The drawing under review shows one solid part. Ordinate dimensions are in mm from its lowest x, y, z. A direction names the side the tool comes from. Give positions to 0.01 mm unless a question says otherwise; leave off trailing zeros. Loops run counter-clockwise (first coordinate to the right, second up) from the corner with the lowest first, then second, coordinate; pieces in that order, holes last. Notation, with made-up numbers: (5.25, 42) - (38.25, 42) arc R8 ccw to (38.25, 55) - close; hole circle Ø7 at (40, -17.5). An arc over 180 degrees is marked (long way). Return JSON: item names as keys, results as strings. Group by question number.
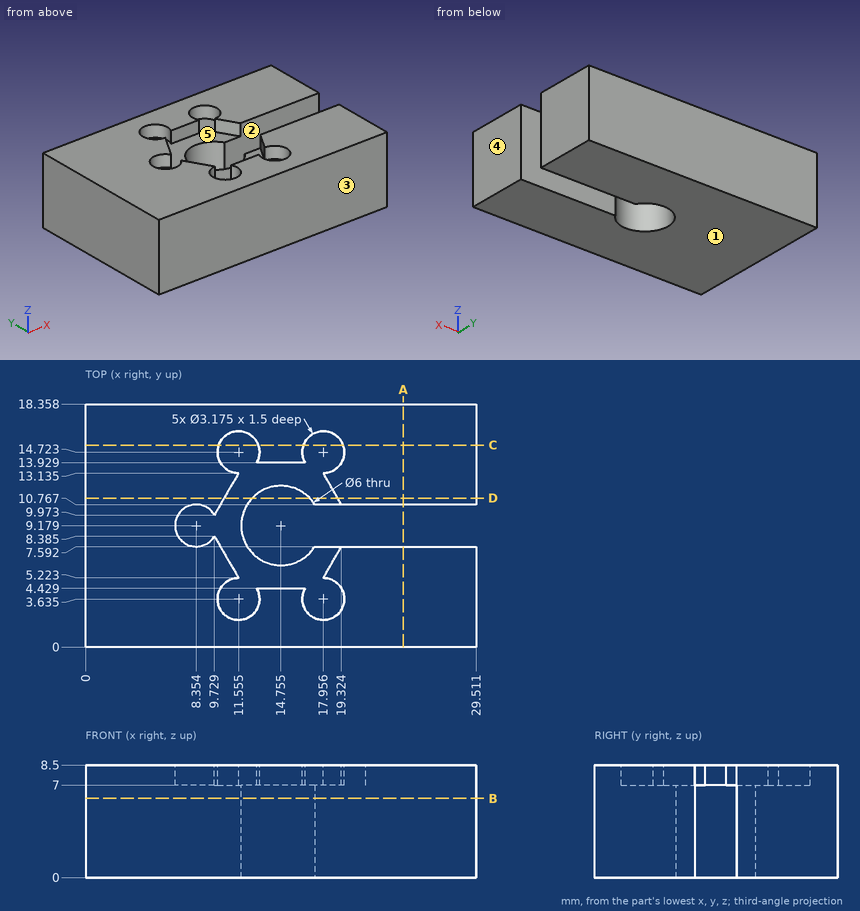
1) We need section B-B, the plane z = 6. Write out the cut boundary in (x, y) (1 decimal).
2) We need section A-A, the plane x = 24. Write out the cut boundary in (y, z).
3) We need section C-C, the plane y = 15.25. Write out the cut boundary in (x, z).
4) Tool access review of the marked faces 1 and 2: name each direction out of +Z, -Z, +X, -X, +Y, -Y from which nothing blocks a thin tool from reaching the whole face with its end or side.
5) Draft analysis for pull direction X (two halves, no side actions). For the marked faces 3, 4 and 5, state which applies: +X half, -X half, draft (parallel to the pull), parting line (faces both ways), or undercut.
6) We need section D-D, the plane y = 11.25. Write out the cut boundary in (x, z) (1 decimal).
7) For pin 1 Ø5.5 at (x, y) = (14.76, 9.18) entering from +Z; pin 2 Ø2.5 at (x, y) = (17.96, 3.64) entering from +Z, all flat-tipped, find the tip position at first contact; note any pin that passes through.
8) To check wall thickness, follow line 1 (X direction, y = 3.75, z = 7.75); line 2 (Y direction, x = 20.75, z = 6.25); line 3 (Y direction, x = 12, z = 4) (1 decimal). State the ranges of each line that lie inside material, in increasing order.
Findings:
{
 "1": {"outline": "(0, 0) - (29.5, 0) - (29.5, 7.6) - (17.3, 7.6) arc R3 cw (long way) to (17.3, 10.8) - (29.5, 10.8) - (29.5, 18.4) - (0, 18.4) - close"},
 "2": {"outline": "(0, 0) - (7.59, 0) - (7.59, 8.5) - (0, 8.5) - close; (10.77, 0) - (18.36, 0) - (18.36, 8.5) - (10.77, 8.5) - close"},
 "3": {"outline": "(0, 0) - (29.51, 0) - (29.51, 8.5) - (19.45, 8.5) - (19.45, 7) - (16.46, 7) - (16.46, 8.5) - (13.05, 8.5) - (13.05, 7) - (10.06, 7) - (10.06, 8.5) - (0, 8.5) - close"},
 "4": {"face 1": "-Z, +X, -X, +Y, -Y", "face 2": "+Z, -Z, +X"},
 "5": {"face 3": "draft", "face 4": "+X half", "face 5": "undercut"},
 "6": {"outline": "(0, 0) - (12.6, 0) - (12.6, 7) - (10.5, 7) - (10.5, 8.5) - (0, 8.5) - close; (16.9, 0) - (29.5, 0) - (29.5, 8.5) - (19, 8.5) - (19, 7) - (16.9, 7) - close"},
 "7": {"pin 1": "passes through", "pin 2": "stops at z = 7"},
 "8": {"line 1": "x = 0 to 9.97, 13.14 to 16.37, 19.54 to 29.51", "line 2": "y = 0 to 7.59, 10.77 to 18.36", "line 3": "y = 0 to 8, 10.4 to 18.4"}
}
